Autodesk Inventor part; units mm, degrees
ref_plane "YZ Plane" through (0, 0, 0) normal (1, 0, 0) x (0, 1, 0)
ref_plane "XZ Plane" through (0, 0, 0) normal (0, 1, 0) x (-1, 0, 0)
ref_plane "XY Plane" through (0, 0, 0) normal (0, 0, 1) x (1, 0, 0)
sketch "Skizze1" plane through (0, 0, 0) normal (0, 0, 1) x (1, 0, 0)
  circle A0 centre (0, 0) radius 72
  circle A1 centre (0, 0) radius 101.5
  circle A2 centre (0, 0) radius 86.75
  dimension "d0" = 144
  dimension "d1" = 203
  dimension "d2" = 29.5
  dimension "d3" = 14.75
extrude "Extrusion1" add sketch "Skizze1" along normal blind 10 contours A1
sketch "Skizze2" plane through (0, 0, 10) normal (0, 0, 1) x (1, 0, 0)
  line L0 (-66.5564, -66.5564) -> (66.5564, -66.5564)
  line L1 (66.5564, -66.5564) -> (66.5564, 66.5564)
  line L2 (66.5564, 66.5564) -> (-66.5564, 66.5564)
  line L3 (-66.5564, 66.5564) -> (-66.5564, -66.5564)
  line L4 (-66.5564, -66.5564) -> (66.5564, 66.5564) construction
  line L5 (66.5564, -66.5564) -> (-66.5564, 66.5564) construction
  circle A0 centre (0, 0) radius 94.125 construction
  circle A1 centre (0, 0) radius 86.75 construction
  circle A2 centre (0, 0) radius 101.5 construction
  dimension "d15" = 14.75
  dimension "d16" = 7.375
hole "Bohrung1" at (-66.5564, 66.5564, 10) at (66.5564, 66.5564, 10) at (66.5564, -66.5564, 10) at (-66.5564, -66.5564, 10) direction (0, 0, -1) diameter 4.9 end through all countersink diameter 9 countersink angle 90
equation "\"d3\" = 0.5 * d2"
equation "\"d16\" = 0.5 * d15"
properties part number "Drehkranz_B" material "ABS-Kunststoff"
The listing builds one solid part. Answer for the finished solid, in the listing's coordinates (mm). Round coordinates to 2 decimals unless told otherwise and drop trailing zeros. Write each loop counter-clockwise with the first axis right and the second up, starting at its lowest first coordinate (ties: lowest second). Pieces come first, ordered by that corner, then holes. Notation, with made-up numbers: (57.5, 10.5) -> (112.5, 10.5) arc R21 cw to (112.5, 33.5) -> close; hole circle Ø11 at (60.25, -14.5). An arc over 180 degrees is marked (long way). Answer as a JSON object with one key per item and string values. Group by question number.
Q1. Section A-A (x = 0) is taken. Write down the section's boundary in (y, z), plus the area to 3 significant figures.
Q2. Section C-C (z = 6) is taken. Write down the section's boundary in (x, y), plus the area to 3 significant figures.
Q3. Determine the mould class of faces 1 (the face through (-68.844, 65.367, 8.078)), 2 (the face through (30, -82, 10)), 3 (the face through (96.813, -30.488, 4.93)) for opening direction Y: pulls with the +Y half, pulls with the -Y half, needs draft (parallel to the pull), parting line crosses it, or undercut.
Q4. Each of these flat-tipped pins is pushed along its axis until it touches: pin 1 Ø3 at (x, z) = (-55, 8) entering from -Y; pin 2 Ø4.5 at (x, y) = (66.56, -66.56) entering from -Z; pin 3 Ø5 at (x, z) = (13.5, 2.5) entering from +Y; pin 4 Ø5 at (x, z) = (34, 2) entering from +Y. Where does it stop, or does it pass through?
Q5. Straight lines are drawn through the part: line 1 along Y through (x, z) = (67, 9.5); line 2 along X through (y, z) = (36.5, 3.5); line 3 along X through (y, z) = (80, 7.75). For each, find the intervals that lie inside material, in ascending order.
Check values:
{
 "1": {"outline": "(-101.5, 0) -> (-86.75, 0) -> (-86.75, 10) -> (-101.5, 10) -> close; (86.75, 0) -> (101.5, 0) -> (101.5, 10) -> (86.75, 10) -> close", "area": "295 mm^2"},
 "2": {"outline": "circle Ø203 at (0, 0); hole circle Ø173.5 at (0, 0); hole circle Ø4.9 at (-66.56, -66.56); hole circle Ø4.9 at (-66.56, 66.56); hole circle Ø4.9 at (66.56, -66.56); hole circle Ø4.9 at (66.56, 66.56)", "area": "8,650 mm^2"},
 "3": {"face 1": "undercut", "face 2": "needs draft", "face 3": "parting line crosses it"},
 "4": {"pin 1": "y = -86.26", "pin 2": "through", "pin 3": "y = 100.9", "pin 4": "y = 96.49"},
 "5": {"line 1": "-76.24 to -70.53, -62.58 to -55.11, 55.11 to 62.58, 70.53 to 76.24", "line 2": "-94.71 to -78.7, 78.7 to 94.71", "line 3": "-62.47 to -33.55, 33.55 to 62.47"}
}
